Autodesk Inventor part; units mm, degrees
ref_plane "Plan de construction1" through (5, 0, 0) normal (-1, 0, 0) x (0, 0, 1)
ref_plane "YZ Plane" through (0, 0, 0) normal (1, 0, 0) x (0, 1, 0)
ref_plane "XZ Plane" through (0, 0, 0) normal (0, 1, 0) x (-1, 0, 0)
sketch "Esquisse1" plane through (0, 0, 0) normal (1, 0, 0) x (0, 1, 0)
  circle A0 centre (0, 0) radius 16
  line L0 (-16, 0) -> (59, 0)
  line L1 (59, 0) -> (51, 0)
  circle A1 centre (51, 0) radius 5
  circle A2 centre (51, 0) radius 8
  line L2 (0, 16) -> (51, 8)
  line L3 (51, -8) -> (0, -16)
  circle A3 centre (0, 0) radius 11
  line L4 (34.396, -10.6045) -> (34.396, 10.6045)
  dimension "d0" = 32
  dimension "d1" = 75
  dimension "d2" = 8
  dimension "d3" = 10
  dimension "d4" = 16
  dimension "d5" = 22
extrude "Extrusion1" add sketch "Esquisse1" along normal blind 10 contours L2 A0 L0 A3 | L0 A3 A0 L3 | L2 L4 L0 A0 | L0 L4 L3 A0
sketch "Esquisse2" plane through (0, 0, 0) normal (-1, 0, 0) x (0, 0, 1)
  circle A0 centre (0, 0) radius 11
  circle A1 centre (0, 0) radius 4.25
  dimension "d8" = 8.5
extrude "Extrusion2" add sketch "Esquisse2" along normal blind 10
sketch "Esquisse3" plane through (-10, 0, 0) normal (-1, 0, 0) x (0, 0, 1)
  line L0 (0, 0) -> (-10, 0)
  circle A0 centre (0, 0) radius 11
  line L1 (0, 0) -> (0, 10)
  circle A1 centre (0, 0) radius 4.25
  line L2 (0, 0) -> (10, 0)
  line L3 (0, 0) -> (0, -10)
  line L4 (0, 10) -> (-10, 0)
  line L5 (0, 10) -> (10, 0)
  line L6 (10, 0) -> (0, -10)
  line L7 (-10, 0) -> (0, -10)
  circle A2 centre (0, 0) radius 4.25
  dimension "d12" = 10
  dimension "d13" = 10
  dimension "d14" = 10
  dimension "d15" = 10
  dimension "d16" = 8.5
extrude "Extrusion3" add sketch "Esquisse3" along normal blind 5 contours A1 L3 L7 L0 | L0 L4 L1 A1 | L1 L5 L2 A1 | L2 L6 L3 A1
sketch "Esquisse4" plane through (0, 0, 0) normal (-1, 0, 0) x (0, 0, 1)
  circle A0 centre (0, 0) radius 13.75
  circle A1 centre (0, 0) radius 11
  dimension "d19" = 27.5
extrude "Extrusion4" add sketch "Esquisse4" along normal up to surface (10 mm away)
ref_plane "Plan de construction1" through (5, 0, 0) normal (-1, 0, 0) x (0, 0, 1)
sketch "Esquisse7" plane through (5, 0, 0) normal (-1, 0, 0) x (0, 0, 1)
  point P0 (0, 0)
sketch "Esquisse8" plane through (5, 0, 0) normal (-1, 0, 0) x (0, 0, 1)
  circle A0 centre (0, 51) radius 5
  circle A1 centre (0, 51) radius 4.25
  line L0 (-16, 0) -> (-10.6045, 34.396)
  line L1 (10.6045, 34.396) -> (16, 0)
  arc A2 (8, 51) -> (-8, 51) centre (0, 51) ccw
  line L2 (-10.6045, 34.396) -> (10.6045, 34.396)
  line L3 (-10.6045, 34.396) -> (-8, 51)
  line L4 (8, 51) -> (10.6045, 34.396)
  line L5 (10.6045, 34.396) -> (-10.6045, 34.396)
  point P0 (0, 0)
extrude "Extrusion6" add sketch "Esquisse8" along normal mid plane 7 contours L4 L2 L3 A2
sketch "Esquisse9" plane through (8.5, 0, 0) normal (1, 0, 0) x (0, 0, -1)
  circle A0 centre (0, 51) radius 5
  circle A1 centre (0, 51) radius 2.75
  circle A2 centre (0, 51) radius 5
  point P0 (0, 0)
  dimension "d37" = 5.5
extrude "Extrusion7" add sketch "Esquisse9" against normal blind 2
fillet "Congé1" radius 10 4 edges at (8.5, 34.396, 0) (1.5, 34.396, 0) (10, 34.396, 0) (0, 34.396, 0)
sketch "Esquisse10" plane through (0, 0, 0) normal (-1, 0, 0) x (0, 0, 1)
  line L0 (-10.9703, 32.0645) -> (10.9703, 32.0645)
  line L1 (-10.9703, 32.0645) -> (10.9703, 32.0645)
  arc A0 (8, 51) -> (-8, 51) centre (0, 51) ccw
  line L2 (-8, 51) -> (-8, 32.0645)
  line L3 (9.7782, 39.6638) -> (8, 51)
  line L4 (8, 51) -> (8, 32.0645)
  arc A1 (8, 51) -> (-8, 51) centre (0, 51) ccw
  line L5 (-10.9703, 32.0645) -> (-8, 51)
  line L6 (8, 51) -> (10.9703, 32.0645)
  point P0 (0, 0)
extrude "Extrusion8" cut sketch "Esquisse10" against normal blind 10 contours L5 L2 L0 | L4 L3 L6 L0
fillet "Congé2" radius 5 2 edges at (5, 32.0645, -8) (5, 32.0645, -10.9703)
fillet "Congé3" radius 5 2 edges at (5, 32.0645, 10.9703) (5, 32.0645, 8)
properties part number "bièlle côté"
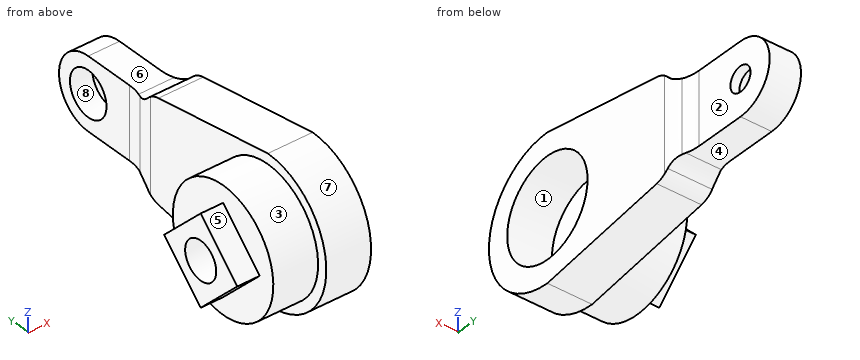
Geometry: final body of the model. Coordinates: model frame, mm. Face numbers are marked on the shaded views. A direction names the side the tool comes from. Coordinates: 2 decimals unless noted, no trailing zeros. Order: outer loops, then holes, each group sorted by start corner. A loop starts at its lowest first (then second) coordinate and runs counter-clockwise, first axis right, second up. Notation, with made-up numbers: (71.5, 16.5) - (97.5, 16.5) arc R25 ccw to (97.5, 44.5) - close; hole circle Ø5 at (73, -6.5). An arc over 180 degrees is marked (long way). Return JSON: item names as keys, results as strings. Group by question number.
1. Cut plane A-A (x = 3.5). Output: boundary loops of the cut face in (y, z).
2. Cut plane B-B (z = -1.5). Count the separate pieces of the cut face and the enclosed holes in it, plus the area to 3 significant figures.
3. Material intervals for line 1 along Y through (x, z) = (7.75, 0); line 2 along Y through (x, z) = (2.95, 0); line 3 along Z through (x, y) = (6.5, 0), sorted ascending. Write a range as [from, to].
4. Pin query (flat end, axial travel): pin 1 (5 mm diameter, centred on x = -4, z = 3.5, fed in from +Y); pin 2 (13.5 mm diameter, centred on y = 0, z = 0, fed in from +X); pin 3 (10 mm diameter, centred on y = 30, z = -4, fed in from -X); pin 4 (3.5 mm diameter, centred on y = 51, z = 0, fed in from -X). Return the tip coordinate at first contact, or that it passes through.
5. Cut plane C-C (x = -10.75). Output: boundary loops of the cut face in (y, z), plus the area to 3 significant figures.
6. Set-up query: the marked faces 1, 2, 3, 4 and 5. Return all of +Z, -Z, +X, -X, +Y, -Y with unobstructed straight access to the full face (end or side cutting, diameter ignored); none if empty.
7. Pull-direction query (Y, two-part tool) for the marked faces 6, 7 and 8; classes: pulls with the +Y half, pulls with the -Y half, needs draft (parallel to the pull), parting line crosses it, or undercut.
8. Cut plane D-D (y = 7). Output: boundary loops of the cut face in (x, z).
Resolved:
{
 "1": {"outline": "(0, -16) - (29.93, -11.31) arc R5 ccw to (32.89, -9.68) arc R5 cw to (36.63, -8) - (51, -8) arc R8 ccw to (51, 8) - (36.63, 8) arc R5 cw to (32.89, 9.68) arc R5 ccw to (29.93, 11.31) - (0, 16) arc R16 ccw to start; hole circle Ø22 at (0, 0); hole circle Ø10 at (51, 0)"},
 "2": {"separate pieces": "3", "enclosed holes": "0", "area": "643 mm²"},
 "3": {"line 1": "y = [-16, -11], [11, 48.25], [53.75, 59]", "line 2": "y = [-16, -11], [11, 46], [56, 59]", "line 3": "z = [-16, -11], [11, 16]"},
 "4": {"pin 1": "stops at y = 13.71", "pin 2": "stops at x = 0", "pin 3": "stops at x = 0", "pin 4": "passes through"},
 "5": {"outline": "(-10, 0) - (0, -10) - (10, 0) - (0, 10) - close; hole circle Ø8.5 at (0, 0)", "area": "143 mm²"},
 "6": {"face 1": "+X", "face 2": "+Z, -Z, +X, +Y", "face 3": "-X", "face 4": "-Z, +X, -X, +Y", "face 5": "+Z, -X, -Y"},
 "7": {"face 6": "needs draft", "face 7": "pulls with the -Y half", "face 8": "undercut"},
 "8": {"outline": "(-15, -3) - (-10, -3) - (-10, -11.83) - (0, -11.83) - (0, -14.9) - (10, -14.9) - (10, -8.49) - (0, -8.49) - (0, 8.49) - (10, 8.49) - (10, 14.9) - (0, 14.9) - (0, 11.83) - (-10, 11.83) - (-10, 3) - (-15, 3) - close"}
}
